from build123d import *


with BuildPart() as part:
    # Sketch1 → Revolve1 (revolve)
    with BuildSketch(Plane.XY, mode=Mode.PRIVATE) as revolve1_sk:
        with BuildLine():
            Line((-7.2, 12.5), (7.2, 12.5))
            ThreePointArc((7.2, 12.5), (7.412132034, 12.587867966), (7.5, 12.8))
            Line((7.5, 12.8), (7.5, 25.7))
            ThreePointArc((7.5, 25.7), (7.412132034, 25.912132034), (7.2, 26))
            Line((7.2, 26), (-7.2, 26))
            ThreePointArc((-7.2, 26), (-7.412132034, 25.912132034), (-7.5, 25.7))
            Line((-7.5, 25.7), (-7.5, 12.8))
            ThreePointArc((-7.5, 12.8), (-7.412132034, 12.587867966), (-7.2, 12.5))
        make_face()
    revolve(revolve1_sk.sketch.rotate(Axis((50, 0, 0), (-1, 0, 0)), 270), axis=Axis((50, 0, 0), (-1, 0, 0)))

    # Sketch2 → Cut-Revolve1 (revolve, cut)
    with BuildSketch(Plane.XY, mode=Mode.PRIVATE) as cut_revolve1_sk:
        Polygon((-9.18, 21.7), (-9.18, 12.5), (-7.5, 12.5), (-7.5, 16.8), (-7.48, 16.8), (-7.48, 19.8), (-7.18, 19.8), (-7.18, 21.7), align=None)
    revolve(cut_revolve1_sk.sketch.rotate(Axis((50, 0, 0), (-1, 0, 0)), 270), axis=Axis((50, 0, 0), (-1, 0, 0)), mode=Mode.SUBTRACT)

    # Sketch3 → Cut-Revolve2 (revolve, cut)
    with BuildSketch(Plane.XY, mode=Mode.PRIVATE) as cut_revolve2_sk:
        Polygon((7.18, 19.8), (7.48, 19.8), (7.48, 16.8), (7.5, 16.8), (7.5, 12.5), (9.18, 12.5), (9.18, 21.7), (7.18, 21.7), align=None)
    revolve(cut_revolve2_sk.sketch.rotate(Axis((50, 0, 0), (-1, 0, 0)), 270), axis=Axis((50, 0, 0), (-1, 0, 0)), mode=Mode.SUBTRACT)


solid = part.part
Could you check a few things on this model? Use its own coordinates, in mm. A direction names the side the tool comes from. Round coordinates to 2 decimals unless told otherwise and drop trailing zeros. Loops run counter-clockwise (first coordinate to the right, second up) from the corner with the lowest first, then second, coordinate; pieces in that order, holes last. Notation, with made-up numbers: (-39.5, 49.25) - (-32.5, 49.25) arc R4 cw to (-32.5, 55.25) - close; hole circle Ø2 at (-33, 49.25). An arc over 180 degrees is marked (long way). Write item = value, one per line.
1) Imagine slicing it at A-A (x = -2.5). Please give me the cut outline in (y, z).
Computed:
outline = circle Ø52 at (0, 0); hole circle Ø25 at (0, 0)
2) If we mould it in two halves opening along Y, with no side actions, what happens to faces 3 (the flat face through (7.18, -10, 18)), 4 (the cylindrical face through (-0.101, -15.821, -20.633)), 5 (the flat face through (-7.5, -12.4, -3.8))? For each: pulls with the +Y half, pulls with the -Y half, needs draft (parallel to the pull), parting line crosses it, or undercut.
Computed:
face_3 = undercut
face_4 = parting line crosses it
face_5 = needs draft
3) I'm going to push flat-ended pins straight in: P1, Ø20, axis at y = 0, z = -3, coming from the -X side; P2, Ø3, axis at x = 4.5, z = 15, coming from the +Y side; P3, Ø2, axis at x = 4, y = 2.5, coming from the +Z side; P4, Ø1, axis at y = 13, z = 13, coming from the +X side. Where does each tip first touch, or does it pass through?
Computed:
P1 = -7.5
P2 = 22.22
P3 = 25.96
P4 = 7.48
4) I need wall thicknesses on line 1 along Y through (x, z) = (7.3, 0); line 2 along Z through (x, y) = (2.25, 0.5); line 3 along Y through (x, z) = (-3.25, 0). Which ranges of each line are inside material? Lowest first, please. Write a range as from..to.
Computed:
line_1 = -25.98..-21.7, -19.8..-12.52, 12.52..19.8, 21.7..25.98
line_2 = -26..-12.49, 12.49..26
line_3 = -26..-12.5, 12.5..26
5) On a 3-axis mill with a long thin cutter (end or side, diameter ignored), from which of +Z, -Z, +X, -X, +Y, -Y can I reach the whole of each face in a straight line? I mean faces 1 (the cylindrical face through (7.338, 6.518, 20.698)), 2 (the flat face through (-7.18, -18, -10)). Say none if no direction works.
Computed:
face_1 = +X
face_2 = -X
